from build123d import *

# Parameters (mm, degrees)
SKETCH1_W                  = 19.05
SKETCH1_H                  = 33.02
BOSS_EXTRUDE1_DEPTH        = 6.35
SKETCH2_R                  = 6.35
BOSS_EXTRUDE2_DEPTH        = 13.462
F_8_0_199_DIAMETER_HOLE1_D = 5.0546
CUT_EXTRUDE1_DEPTH         = 2.54
SKETCH7_R                  = 9.525
SKETCH7_R_2                = 6.35
BOSS_EXTRUDE3_DEPTH        = 7.874
CUT_EXTRUDE2_START         = -3.048
CUT_EXTRUDE2_DEPTH         = 3.048
FILLET1_R                  = 9.525


with BuildPart() as part:
    # Sketch1 → Boss-Extrude1 (new body)
    with BuildSketch(Plane.XY):
        with Locations((0, 16.51)):
            Rectangle(SKETCH1_W, SKETCH1_H)
    extrude(amount=BOSS_EXTRUDE1_DEPTH)

    # Sketch2 → Boss-Extrude2 (add)
    with BuildSketch(Plane.XY.offset(6.35)):
        with Locations(Location((0, 9.525, 0), (0, 0, 180))):
            Circle(SKETCH2_R)
    extrude(amount=BOSS_EXTRUDE2_DEPTH)

    # #8 (0.199) Diameter Hole1 (through all)
    with Locations(Plane.XY.offset(19.812)):
        with Locations((0, 9.525)):
            Hole(F_8_0_199_DIAMETER_HOLE1_D / 2)

    # Sketch5 → Cut-Extrude1 (cut)
    with BuildSketch(Plane(origin=(0, 0, 0), x_dir=(-1, 0, 0), z_dir=(0, 0, -1))):
        Polygon((2.346351494, 5.461), (4.692702988, 9.525), (2.346351494, 13.589), (-2.346351494, 13.589), (-4.692702988, 9.525), (-2.346351494, 5.461), align=None)
    extrude(amount=-CUT_EXTRUDE1_DEPTH, mode=Mode.SUBTRACT)

    # Sketch7 → Boss-Extrude3 (add)
    with BuildSketch(Plane.XY.offset(6.35)):
        with Locations((0, 9.525)):
            Circle(SKETCH7_R)
        with Locations((0, 9.525)):
            Circle(SKETCH7_R_2, mode=Mode.SUBTRACT)
    extrude(amount=BOSS_EXTRUDE3_DEPTH)

    # Sketch8 → Cut-Extrude2 (cut)
    with BuildSketch(Plane.XY.offset(19.812).offset(CUT_EXTRUDE2_START)):
        with BuildLine():
            Line((1.53852276, 11.530041897), (3.865635074, 14.562793711))
            ThreePointArc((3.865635074, 14.562793711), (0, 15.875), (-3.865635074, 14.562793711))
            Line((-3.865635074, 14.562793711), (-1.53852276, 11.530041897))
            ThreePointArc((-1.53852276, 11.530041897), (0, 12.0523), (1.53852276, 11.530041897))
        make_face()
    extrude(amount=CUT_EXTRUDE2_DEPTH, mode=Mode.SUBTRACT)

    # Fillet1
    fillet1_edges = [part.edges().sort_by_distance(p)[0] for p in [
        (9.525, 0, 3.175),
        (-9.525, 0, 3.175),
        (9.525, 33.02, 3.175),
        (-9.525, 33.02, 3.175),
    ]]
    fillet(fillet1_edges, radius=FILLET1_R - 0.0001)  # a hair under: the kernel refuses the full size


solid = part.part
Read the model definition and answer for the solid it produces. Units are mm, in the model's axes. A direction names the side the tool comes from. Give positions to 0.01 mm unless a question says otherwise; leave off trailing zeros. Return JSON: item names as keys, results as strings.
Q1. For faces 1 (the face through (-2.72, 13.07, 18.27)), 2 (the face through (9.525, 16, 3)), 3 (the face through (0.83, 3.23, 16.98)), 4 (the face through (-3.5, 7.46, 1.25)), determine the directions among +Z, -Z, +X, -X, +Y, -Y from which every point of the face is accessible in a straight line to the end or side of a thin tool.
Reply:
{"face 1": "+Z, +Y", "face 2": "+Z, -Z, +X, +Y, -Y", "face 3": "+Z", "face 4": "-Z"}
Q2. Given P1, Ø2, axis at y = 21, z = 9, coming from the +X side; P2, Ø8, axis at x = 0, y = 9.525, coming from the -Z side; P3, Ø5, axis at x = 4.5, z = 3, coming from the -Y side; P4, Ø3.5, axis at x = -1, y = 14.5, coming from the +Z side, each flat-ended and moving along its own axis, determine where each tip first touches the part or whether it passes through.
Reply:
{"P1": "through", "P2": "z = 2.54", "P3": "y = 0.21", "P4": "z = 16.76"}
Q3. For a pull along X with two mould halves and no side action, classify faces 5 (the face through (6.809, 2.864, 3.219)), 6 (the face through (0, 24, 6.35)), 7 (the face through (3.536, 7.521, 1.252)) as released by +X, released by -X, zero draft, split by the parting line, or undercut.
Reply:
{"face 5": "released by +X", "face 6": "zero draft", "face 7": "undercut"}
Q4. Consider line 1 along Y through (x, z) = (0, 16.5) (3 decimals); line 2 along Y through (x, z) = (0, 12.5); line 3 along Z through (x, y) = (3.25, 19.5). Determine where each line is inside the solid, lowest interval first. Write a range as [from, to].
Reply:
{"line 1": "[3.175, 6.998], [12.052, 15.875]", "line 2": "[0, 7], [12.05, 19.05]", "line 3": "[0, 6.35]"}
